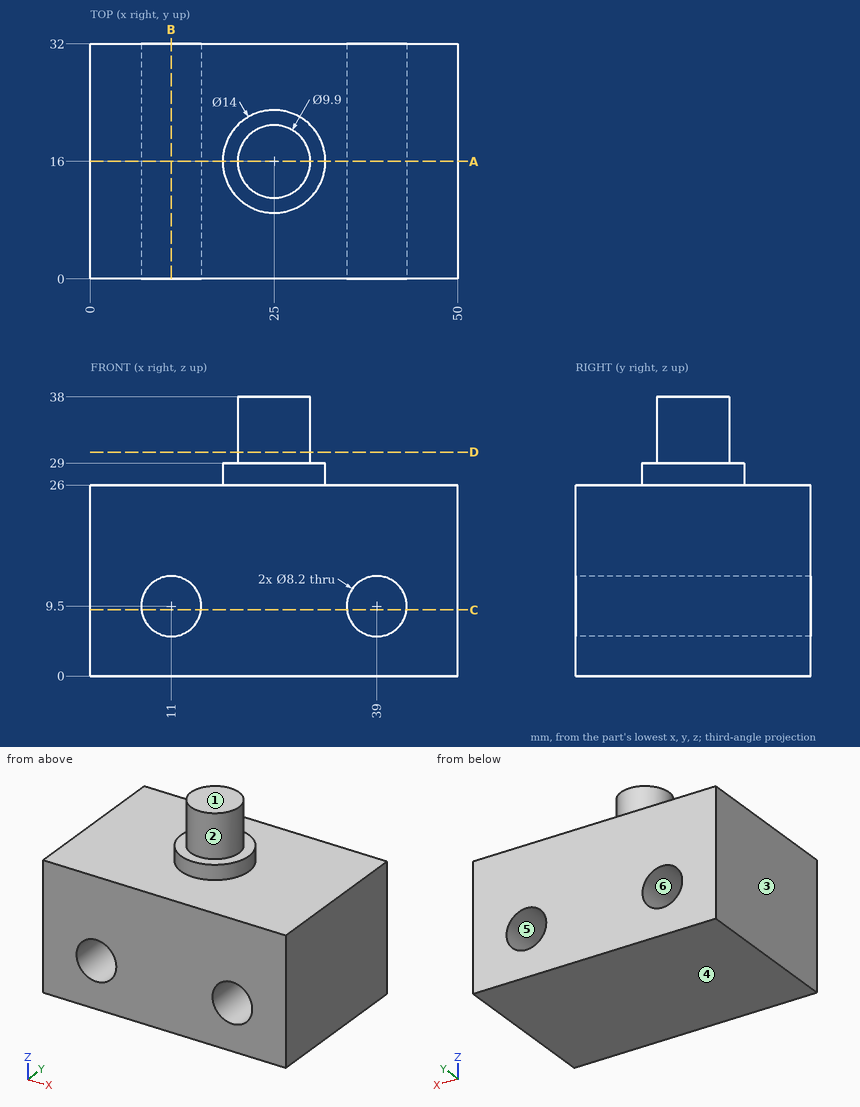
Could you check a few things on this drawing? It's one solid part, dimensions in mm from its lowest x, y, z. A direction names the side the tool comes from. Round coordinates to 2 decimals unless told otherwise and drop trailing zeros. Loops run counter-clockwise (first coordinate to the right, second up) from the corner with the lowest first, then second, coordinate; pieces in that order, holes last. Notation, with made-up numbers: (27, -11.75) -> (73, -11.75) arc R27 cw to (73, 5.25) -> close; hole circle Ø9 at (-28, 55). An arc over 180 degrees is marked (long way). One line per item, written item: value. Start each with the question number.
1. If we section it at C-C, the plane z = 9: Write out the boundary of the cut face in (x, y), then the cut area to 3 significant figures.
2. If we section it at D-D, the plane z = 30.5: Write out the boundary of the cut face in (x, y), then the cut area to 3 significant figures.
3. If we section it at B-B, the plane x = 11: Write out the boundary of the cut face in (y, z).
4. For the marked faces 1 and 2, which set-ups out of +Z, -Z, +X, -X, +Y, -Y let a thin tool reach every point of the face, with its end or its side?
5. If we section it at A-A, the plane y = 16: Write out the boundary of the cut face in (x, z), then the cut area to 3 significant figures.
6. For pin 1 (4 mm diameter, centred on x = 23.5, y = 24, fed in from +Z); pin 2 (6 mm diameter, centred on x = 15.5, y = 26.5, fed in from +Z); pin 3 (5 mm diameter, centred on x = 11, z = 9.5, fed in from +Y), each with a flat end and sliding along its axis, tell me the tip position at first contact or that it passes through.
7. If we mould it in two halves opening along X, with no side actions, what happens to the marked faces 3, 4, 5 and 6? For each: pulls with the +X half, pulls with the -X half, needs draft (parallel to the pull), parting line crosses it, or undercut.
8. If I drill on probe 1 along X at (y, z) = (18.5, 9.5); probe 2 along Z at (x, y) = (39, 20); probe 3 along X at (y, z) = (2.5, 10.5), over which ranges is the centre line in solid material (lowest first)?
Calculated:
1. outline: (0, 0) -> (6.93, 0) -> (6.93, 32) -> (0, 32) -> close; (15.07, 0) -> (34.93, 0) -> (34.93, 32) -> (15.07, 32) -> close; (43.07, 0) -> (50, 0) -> (50, 32) -> (43.07, 32) -> close
1. area: 1,080 mm²
2. outline: circle Ø9.9 at (25, 16)
2. area: 77.0 mm²
3. outline: (0, 0) -> (32, 0) -> (32, 5.4) -> (0, 5.4) -> close; (0, 13.6) -> (32, 13.6) -> (32, 26) -> (0, 26) -> close
4. face 1: +Z, +X, -X, +Y, -Y
4. face 2: +Z
5. outline: (0, 0) -> (50, 0) -> (50, 26) -> (32, 26) -> (32, 29) -> (29.95, 29) -> (29.95, 38) -> (20.05, 38) -> (20.05, 29) -> (18, 29) -> (18, 26) -> (0, 26) -> close; hole circle Ø8.2 at (11, 9.5); hole circle Ø8.2 at (39, 9.5)
5. area: 1,330 mm²
6. pin 1: stops at z = 29
6. pin 2: stops at z = 26
6. pin 3: passes through
7. face 3: pulls with the -X half
7. face 4: needs draft
7. face 5: undercut
7. face 6: undercut
8. probe 1: x = 0 to 6.9, 15.1 to 34.9, 43.1 to 50
8. probe 2: z = 0 to 5.4, 13.6 to 26
8. probe 3: x = 0 to 7.02, 14.98 to 35.02, 42.98 to 50
